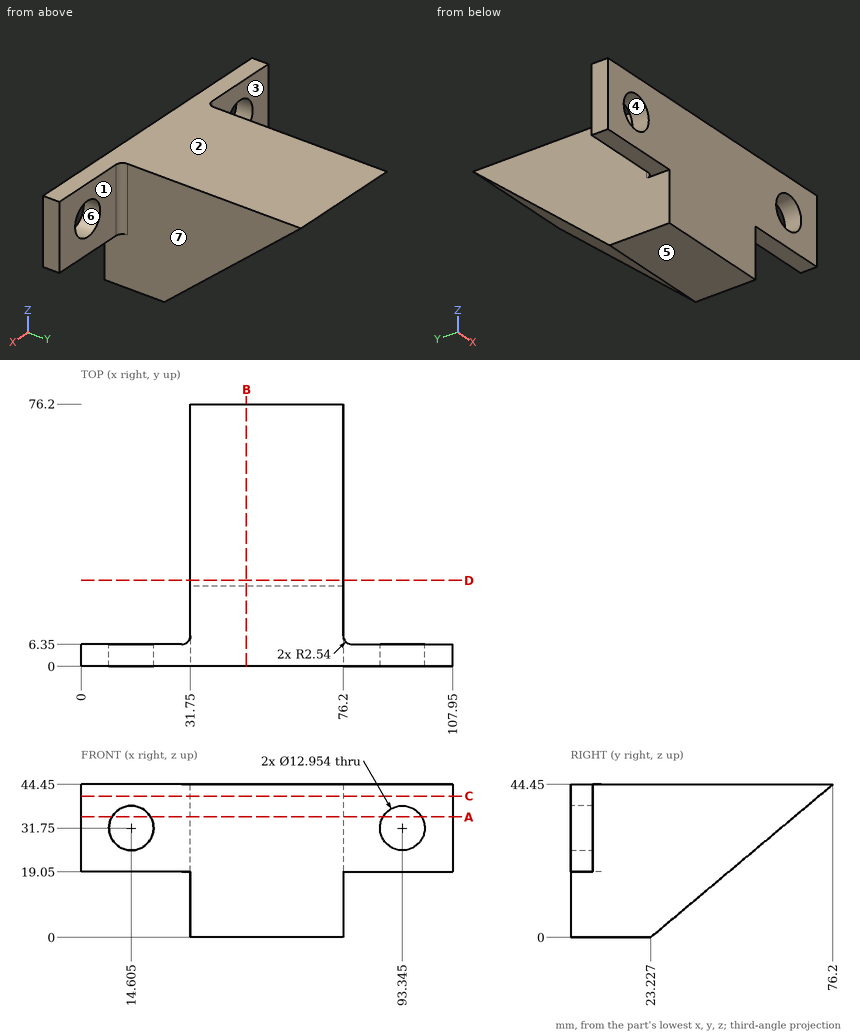
Geometry check sheet. Reference: drawing and pictorial views, mm from the part's lowest x, y, z. A direction names the side the tool comes from. Coordinates: 2 decimals unless noted, no trailing zeros. Write each loop counter-clockwise with the first axis right and the second up, starting at its lowest first coordinate (ties: lowest second). Pieces come first, ordered by that corner, then holes.
Item 1: Mould release check, pull along Z, two halves, no side actions. Record for the marked faces 4, 5, 6 and 7: released by +Z, released by -Z, zero draft, split by the parting line, or undercut.
Numbers:
face 4: undercut
face 5: released by -Z
face 6: undercut
face 7: zero draft
Item 2: Cross-section at D-D on y = 25. Record the boundary of the cut face in (x, z), then the cut area to 3 significant figures.
Numbers:
outline: (31.75, 1.49) - (76.2, 1.49) - (76.2, 44.45) - (31.75, 44.45) - close
area: 1,910 mm2
Item 3: Depth check by flat-ended pin: pin 1 Ø22 at (y, z) = (37, 31) entering from -X; pin 2 Ø20.5 at (x, z) = (88.5, 30) entering from +Y; pin 3 Ø2 at (x, z) = (87.5, 39.5) entering from +Y. Enter the tip coordinate at first touch or a pass-through.
Numbers:
pin 1: stops at x = 31.75
pin 2: stops at y = 6.4
pin 3: stops at y = 6.35
Item 4: Access from +Z, -Z, +X, -X, +Y, -Y to the whole of each face (thin tool, end or side, straight path). Record for the marked faces 1, 2 and 3.
Numbers:
face 1: +Z, -Z, +X, +Y
face 2: +Z, +X, -X, +Y, -Y
face 3: +Z, -Z, -X, +Y
Item 5: Cross-section at A-A on z = 35. Record the boundary of the cut face in (x, y), then the cut area to 3 significant figures.
Numbers:
outline: (0, 0) - (9, 0) - (9, 6.35) - (0, 6.35) - close; (20.21, 0) - (87.74, 0) - (87.74, 6.35) - (78.74, 6.35) arc R2.54 cw to (76.2, 8.89) - (76.2, 64.94) - (31.75, 64.94) - (31.75, 8.89) arc R2.54 cw to (29.21, 6.35) - (20.21, 6.35) - close; (98.95, 0) - (107.95, 0) - (107.95, 6.35) - (98.95, 6.35) - close
area: 3,150 mm2
Item 6: Cross-section at C-C on z = 41. Record the boundary of the cut face in (x, y).
Numbers:
outline: (0, 0) - (107.95, 0) - (107.95, 6.35) - (78.74, 6.35) arc R2.54 cw to (76.2, 8.89) - (76.2, 72.09) - (31.75, 72.09) - (31.75, 8.89) arc R2.54 cw to (29.21, 6.35) - (0, 6.35) - close
Item 7: Scan lines: probe 1 along X at (y, z) = (3.75, 31.75); probe 2 along X at (y, z) = (2, 31); probe 3 along Y at (x, z) = (25, 32). Record each from-to range of solid material in increasing order.
Numbers:
probe 1: x = 0 to 8.13, 21.08 to 86.87, 99.82 to 107.95
probe 2: x = 0 to 8.17, 21.04 to 86.91, 99.78 to 107.95
probe 3: y = 0 to 6.35
Item 8: Cross-section at B-B on x = 48. Record the boundary of the cut face in (y, z).
Numbers:
outline: (0, 0) - (23.23, 0) - (76.2, 44.45) - (0, 44.45) - close
